Source: three-view drawing plus pictorial views. Frame: mm from the lowest corner of the part. A direction names the side the tool comes from. Round coordinates to 2 decimals unless told otherwise and drop trailing zeros. Loops run counter-clockwise (first coordinate to the right, second up) from the corner with the lowest first, then second, coordinate; pieces in that order, holes last. Notation, with made-up numbers: M -38.75,75.25 L -2.75,75.25 A25 ccw -2.75,110.25 Z; hole C 87.25,4 d2. An arc over 180 degrees is marked long. Return JSON: item names as keys, results as strings. Group by question number.
1) Section A-A (y = 13.5). Output: boundary loops of the cut face in (x, z), plus the area to 3 significant figures.
2) Material intervals for line 1 (Z direction, x = 7.5, y = 15.75); line 2 (Z direction, x = 7.5, y = 0.1); line 3 (Z direction, x = 7.5, y = 0.2), sorted ascending. Write a range as from..to.
3) Contact query for flat-ended pins moving along their axis: P1, Ø5, axis at x = 10.5, y = 7, coming from the -Z side; P2, Ø5, axis at x = 2, y = 12, coming from the -Z side; P3, Ø4, axis at x = 13, y = 16, coming from the +Z side. Output: stop coordinate, or through.
4) Access query for the marked faces 1 and 2. Directions: +Z, -Z, +X, -X, +Y, -Y. A direction counts if a zero-diameter tool reaches every point of the face in a straight line with its end or side. Return the directions, or none.
5) Mould query, pull axis X, two halves, no side actions, for the marked faces 3, 4 and 5. Classes: +X half, -X half, draft (parallel to the pull), parting line (faces both ways), or undercut.
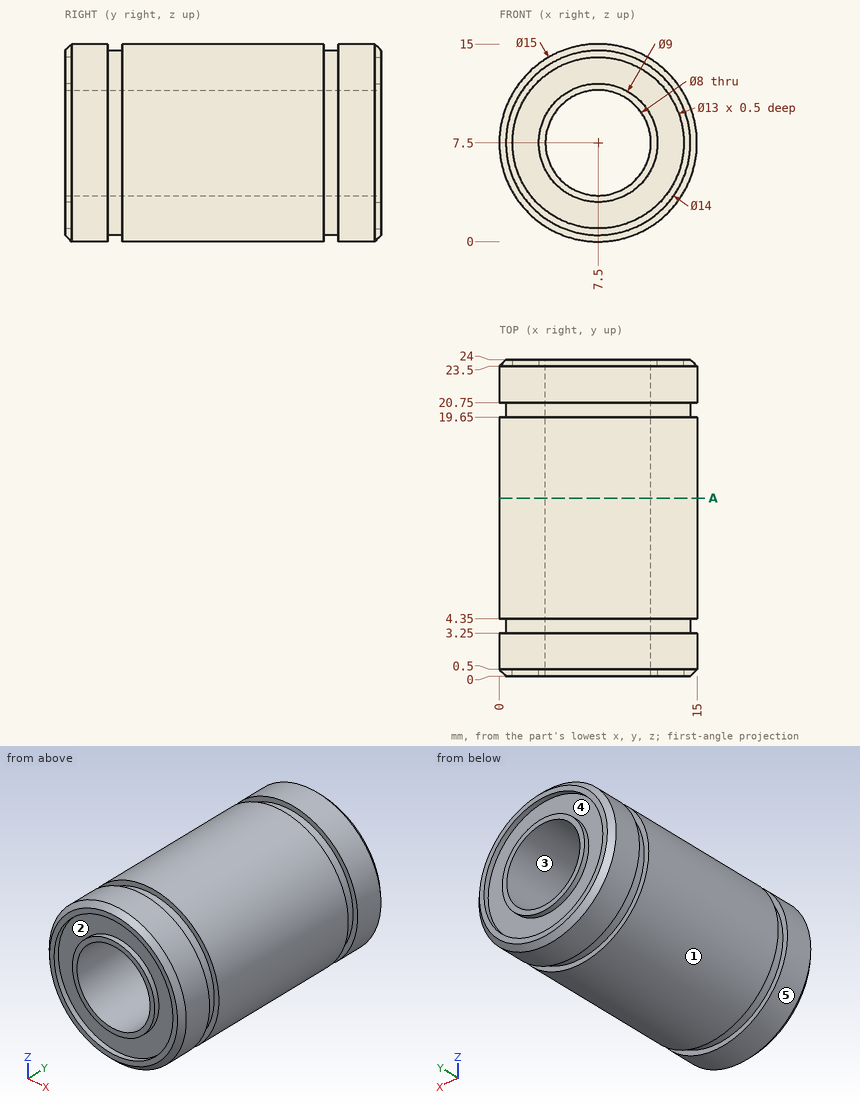
Returned:
{
 "1": {"outline": "C 7.5,7.5 d15; hole C 7.5,7.5 d8", "area": "126 mm^2"},
 "2": {"line 1": "z = 0..3.5, 11.5..15", "line 2": "z = 0.4..1, 3..3.5, 11.5..12, 14..14.6", "line 3": "z = 0.3..1, 3..3.5, 11.5..12, 14..14.7"},
 "3": {"P1": "stops at z = 0.02", "P2": "stops at z = 0.63", "P3": "stops at z = 14.13"},
 "4": {"face 1": "+Y, -Y", "face 2": "-Y"},
 "5": {"face 3": "undercut", "face 4": "undercut", "face 5": "parting line"}
}
